from build123d import *

# Parameters (mm, degrees)
EXTRUDE_1_DEPTH     = 12
SKETCH_2_R          = 2
CUT_EXTRUDE_1_DEPTH = 12
SKETCH_3_R          = 2
CUT_EXTRUDE_2_DEPTH = 12


with BuildPart() as part:
    # 草图1 → 凸台-拉伸1 (new body)
    with BuildSketch(Plane(origin=(0, 0, 0), x_dir=(0, 0, -1), z_dir=(1, 0, 0))):
        Polygon((0, 0), (61, 0), (61, 1.2), (1.2, 1.2), (1.2, 61), (0, 61), align=None)
    extrude(amount=EXTRUDE_1_DEPTH)

    # 草图2 → 切除-拉伸1 (cut)
    with BuildSketch(Plane(origin=(0, 1.2, 0), x_dir=(1, 0, 0), z_dir=(0, 1, 0))):
        with Locations(Location((6, 21.2, 0), (0, 0, 270))):
            Circle(SKETCH_2_R)
        with Locations(Location((6, 53.2, 0), (0, 0, 270))):
            Circle(SKETCH_2_R)
    extrude(amount=-CUT_EXTRUDE_1_DEPTH, mode=Mode.SUBTRACT)

    # 草图3 → 切除-拉伸2 (cut)
    with BuildSketch(Plane(origin=(0, 0, -1.2), x_dir=(-1, 0, 0), z_dir=(0, 0, -1))):
        with Locations(Location((-6, 21.2, 0), (0, 0, 90))):
            Circle(SKETCH_3_R)
        with Locations(Location((-6, 53.2, 0), (0, 0, 90))):
            Circle(SKETCH_3_R)
    extrude(amount=-CUT_EXTRUDE_2_DEPTH, mode=Mode.SUBTRACT)


solid = part.part
The model under review builds one solid part; all positions refer to its coordinate system, in mm. A direction names the side the tool comes from. Coordinates: 2 decimals unless noted, no trailing zeros. Write each loop counter-clockwise with the first axis right and the second up, starting at its lowest first coordinate (ties: lowest second). Pieces come first, ordered by that corner, then holes. Notation, with made-up numbers: M 51,-3.5 L 74,-3.5 A29 cw 74,27.5 Z; hole C 80.25,12 d9. An arc over 180 degrees is marked long. Put each result on its own line as item: value.
1) Clearance check with flat-ended pins moving along their axes: pin 1 Ø4 at (x, z) = (4, -45.5) entering from +Y; pin 2 Ø4 at (x, y) = (4.5, 20) entering from -Z. State where each tip first meets the part, or that it passes through.
Computed:
pin 1: stops at y = 1.2
pin 2: stops at z = -1.2
2) Add section D-D on x = 11.25. Give the boundary of the cut face in (y, z), then the cut area to 3 significant figures.
Computed:
outline: M 0,-61 L 1.2,-61 L 1.2,-1.2 L 61,-1.2 L 61,0 L 0,0 Z
area: 145 mm2
3) Draft analysis for pull direction Y (two halves, no side actions). For faces 3 (the cylindrical face through (6.601, 23.108, -0.608)), 4 (the flat face through (6, 1.2, -32)), 5 (the cylindrical face through (6.601, 0.608, -51.292)), 6 (the flat face through (6, 0, -30)), state which applies: released by +Y, released by -Y, zero draft, split by the parting line, or undercut.
Computed:
face 3: undercut
face 4: released by +Y
face 5: zero draft
face 6: released by -Y
4) Add section B-B on z = -53.2. Give the boundary of the cut face in (x, y).
Computed:
outline: M 0,0 L 4,0 L 4,1.2 L 0,1.2 Z; M 8,0 L 12,0 L 12,1.2 L 8,1.2 Z
5) Wall thickness on probe 1 along X at (y, z) = (0.9, -53.2); probe 2 along Y at (x, z) = (1, -16); probe 3 along Z at (x, y) = (8.75, 46): over which ranges is each line inside the solid? List them lowest first. Write a range as [from, to].
Computed:
probe 1: x = [0, 4], [8, 12]
probe 2: y = [0, 1.2]
probe 3: z = [-1.2, 0]
6) Add section A-A on x = 6. Give the boundary of the cut face in (y, z), then the cut area to 3 significant figures.
Computed:
outline: M 0,-61 L 1.2,-61 L 1.2,-55.2 L 0,-55.2 Z; M 0,-51.2 L 1.2,-51.2 L 1.2,-23.2 L 0,-23.2 Z; M 0,-19.2 L 1.2,-19.2 L 1.2,-1.2 L 19.2,-1.2 L 19.2,0 L 0,0 Z; M 23.2,-1.2 L 51.2,-1.2 L 51.2,0 L 23.2,0 Z; M 55.2,-1.2 L 61,-1.2 L 61,0 L 55.2,0 Z
area: 126 mm2
7) Add section C-C on y = 53.2. Give the boundary of the cut face in (x, z), then the cut area to 3 significant figures.
Computed:
outline: M 0,-1.2 L 4,-1.2 L 4,0 L 0,0 Z; M 8,-1.2 L 12,-1.2 L 12,0 L 8,0 Z
area: 9.60 mm2
8) For faces 1 (the flat face through (6, 31, -1.2)), 2 (the flat face through (6, 31, 0)), list the 3-axis set-ups (+Z, -Z, +X, -X, +Y, -Y) from which the entire face can be reached by the end or side of a thin tool; tool diameter is ignored.
Computed:
face 1: -Z, +X, -X, +Y
face 2: +Z, +X, -X, +Y, -Y
